from build123d import *

# Parameters (mm, degrees)
CROQUIS1_W                 = 20
CROQUIS1_H                 = 15
SALIENTE_EXTRUIR1_DEPTH    = 100
CROQUIS2_W                 = 16
CROQUIS2_H                 = 13
CORTAR_EXTRUIR2_DEPTH      = 100
CROQUIS3_R                 = 4.15
CORTAR_EXTRUIR3_DEPTH      = 2
CORTAR_EXTRUIR5_DEPTH      = 103.255806681
CORTAR_EXTRUIR5_DEPTH_BACK = 103.255806681
CROQUIS4_R                 = 1.75


with BuildPart() as part:
    # Croquis1 → Saliente-Extruir1 (new body)
    with BuildSketch(Plane.XY):
        Rectangle(CROQUIS1_W, CROQUIS1_H)
    extrude(amount=SALIENTE_EXTRUIR1_DEPTH)

    # Croquis2 → Cortar-Extruir2 (cut)
    with BuildSketch(Plane(origin=(0, 0, 0), x_dir=(-1, 0, 0), z_dir=(0, 0, -1))):
        with Locations((0, -1)):
            Rectangle(CROQUIS2_W, CROQUIS2_H)
    extrude(amount=-CORTAR_EXTRUIR2_DEPTH, mode=Mode.SUBTRACT)

    # Croquis3 → Cortar-Extruir3 (cut)
    with BuildSketch(Plane(origin=(0, 7.5, 0), x_dir=(1, 0, 0), z_dir=(0, 1, 0))):
        with Locations(Location((3.5, -5.419128069, 0), (0, 0, 270))):
            Circle(CROQUIS3_R)
        with Locations(Location((-3.5, -13.419128069, 0), (0, 0, 270))):
            Circle(CROQUIS3_R)
        with Locations(Location((3.5, -21.419128069, 0), (0, 0, 270))):
            Circle(CROQUIS3_R)
        with Locations(Location((-3.5, -29.419128069, 0), (0, 0, 270))):
            Circle(CROQUIS3_R)
        with Locations(Location((3.5, -37.419128069, 0), (0, 0, 270))):
            Circle(CROQUIS3_R)
        with Locations(Location((-3.5, -45.419128069, 0), (0, 0, 270))):
            Circle(CROQUIS3_R)
        with Locations(Location((3.5, -53.419128069, 0), (0, 0, 270))):
            Circle(CROQUIS3_R)
        with Locations(Location((-3.5, -61.419128069, 0), (0, 0, 270))):
            Circle(CROQUIS3_R)
        with Locations(Location((3.5, -69.419128069, 0), (0, 0, 270))):
            Circle(CROQUIS3_R)
        with Locations(Location((-3.5, -77.419128069, 0), (0, 0, 270))):
            Circle(CROQUIS3_R)
        with Locations(Location((3.5, -85.419128069, 0), (0, 0, 270))):
            Circle(CROQUIS3_R)
        with Locations(Location((-3.5, -93.419128069, 0), (0, 0, 270))):
            Circle(CROQUIS3_R)
    extrude(amount=-CORTAR_EXTRUIR3_DEPTH, mode=Mode.SUBTRACT)

    # Croquis4 → Cortar-Extruir5 (cut, two sides: drawn at the far end of the back side and taken through both)
    with BuildSketch(Plane(origin=(10, 0, 0), x_dir=(0, 0, -1), z_dir=(1, 0, 0)).offset(-CORTAR_EXTRUIR5_DEPTH_BACK)):
        with Locations((-32.5, -2.8)):
            Circle(CROQUIS4_R)
        with Locations((-47.5, -2.8)):
            Circle(CROQUIS4_R)
    extrude(amount=CORTAR_EXTRUIR5_DEPTH + CORTAR_EXTRUIR5_DEPTH_BACK, mode=Mode.SUBTRACT)


solid = part.part
Model file for the job. Use its own axes, mm. A direction names the side the tool comes from. Round coordinates to 2 decimals unless told otherwise and drop trailing zeros. Loops run counter-clockwise (first coordinate to the right, second up) from the corner with the lowest first, then second, coordinate; pieces in that order, holes last. Notation, with made-up numbers: (85, 41) - (110, 41) arc R33 cw to (110, 72) - close; hole circle Ø8 at (59, 83). An arc over 180 degrees is marked (long way). Write each question's results on one line, items separated by ' | '.
(1) Saw through at B-B, the plane x = 3.5. List the corners of the cut face in (y, z), then the cut area to 3 significant figures.
Answer below:
outline: (5.5, 0) - (7.5, 0) - (7.5, 1.27) - (5.5, 1.27) - close; (5.5, 9.57) - (7.5, 9.57) - (7.5, 17.27) - (5.5, 17.27) - close; (5.5, 25.57) - (7.5, 25.57) - (7.5, 33.27) - (5.5, 33.27) - close; (5.5, 41.57) - (7.5, 41.57) - (7.5, 49.27) - (5.5, 49.27) - close; (5.5, 57.57) - (7.5, 57.57) - (7.5, 65.27) - (5.5, 65.27) - close; (5.5, 73.57) - (7.5, 73.57) - (7.5, 81.27) - (5.5, 81.27) - close; (5.5, 89.57) - (7.5, 89.57) - (7.5, 100) - (5.5, 100) - close | area: 100 mm^2
(2) Saw through at C-C, the plane z = 59. List the corners of the cut face in (x, y), then the cut area to 3 significant figures.
Answer below:
outline: (-10, -7.5) - (-8, -7.5) - (-8, 5.5) - (-6.87, 5.5) - (-6.87, 7.5) - (-10, 7.5) - close; (-0.13, 5.5) - (8, 5.5) - (8, -7.5) - (10, -7.5) - (10, 7.5) - (-0.13, 7.5) - close | area: 78.5 mm^2
(3) Wall check: L1, parallel to Z at x = -8.4, y = -2.8; L2, parallel to X at y = -1.5, z = 81; L3, parallel to Y at x = -8.45, z = 47.5. Give the ranges that are in metal, low to high.
Answer below:
L1: z = 0 to 30.75, 34.25 to 45.75, 49.25 to 100 | L2: x = -10 to -8, 8 to 10 | L3: y = -7.5 to -4.55, -1.05 to 7.5
(4) Saw through at A-A, the plane y = -2.8. List the corners of the cut face in (x, z), then the cut area to 3 significant figures.
Answer below:
outline: (-10, 0) - (-8, 0) - (-8, 30.75) - (-10, 30.75) - close; (-10, 34.25) - (-8, 34.25) - (-8, 45.75) - (-10, 45.75) - close; (-10, 49.25) - (-8, 49.25) - (-8, 100) - (-10, 100) - close; (8, 0) - (10, 0) - (10, 30.75) - (8, 30.75) - close; (8, 34.25) - (10, 34.25) - (10, 45.75) - (8, 45.75) - close; (8, 49.25) - (10, 49.25) - (10, 100) - (8, 100) - close | area: 372 mm^2
(5) 3-axis set-ups, long thin cutter, end or side, ignore diameter. For faces 1 (the flat face through (-8, -1, 49)), 2 (the flat face through (0, 6, 0)): which of +Z, -Z, +X, -X, +Y, -Y reach the whole face in a straight line?
Answer below:
face 1: +Z, -Z, -Y | face 2: -Z, +X, -X, +Y, -Y
(6) Saw through at D-D, the plane z = 32. List the corners of the cut face in (x, y).
Answer below:
outline: (-10, -7.5) - (-8, -7.5) - (-8, -4.48) - (-10, -4.48) - close; (-10, -1.12) - (-8, -1.12) - (-8, 5.5) - (-6.75, 5.5) - (-6.75, 7.5) - (-10, 7.5) - close; (-0.25, 5.5) - (8, 5.5) - (8, -1.12) - (10, -1.12) - (10, 7.5) - (-0.25, 7.5) - close; (8, -7.5) - (10, -7.5) - (10, -4.48) - (8, -4.48) - close
(7) Pin check, flat tip, straight feed: pin 1 (5.5 mm diameter, centred on y = -2.8, z = 47.5, fed in from +X). Stop position of the tip, or through.
Answer below:
pin 1: stops at x = 10
(8) Mould opens along X. For faces 3 (the cylindrical face through (8.99, -2.72, 34.25)), 4 (the flat face through (10, 0, 49)), 5 (the flat face through (8, -1, 49)) say: released by +X, released by -X, zero draft, split by the parting line, or undercut.
Answer below:
face 3: zero draft | face 4: released by +X | face 5: undercut
